```python
from build123d import *

# Parameters (mm, degrees)
F0_W     = 508
F0_H     = 508
F1_DEPTH = 15.875
F4_R     = 12.7
F5_R     = 12.7
F6_R     = 12.7


# Not quite as in the source:
# - the program builds the solid bodies; features that only make, move or delete a surface that nothing else refers to are left out


with BuildPart() as f1:
    # F0 (on Top) → F1 (new body)
    with BuildSketch(Plane.XY):
        with Locations((-1.661028713, -10.90797159)):
            Rectangle(F0_W, F0_H)
    extrude(amount=F1_DEPTH)

    # F4
    f4_edges = [f1.edges().sort_by_distance(p)[0] for p in [
        (252.338971, 243.092028, 7.9375),
        (252.338971, -264.907972, 7.9375),
    ]]
    fillet(f4_edges, radius=F4_R)

    # F5
    f5_edges = [f1.edges().sort_by_distance(p)[0] for p in [
        (-255.661029, 243.092028, 7.9375),
        (-255.661029, -264.907972, 7.9375),
    ]]
    fillet(f5_edges, radius=F5_R)

    # F6
    f6_edges = [f1.edges().sort_by_distance(p)[0] for p in [
        (-1.661029, 243.092028, 15.875),
        (-251.941285, 239.372285, 15.875),
        (248.619227, 239.372285, 15.875),
        (-255.661029, -10.907972, 15.875),
        (252.338971, -10.907972, 15.875),
        (-251.941285, -261.188228, 15.875),
        (248.619227, -261.188228, 15.875),
        (-1.661029, -264.907972, 15.875),
    ]]
    fillet(f6_edges, radius=F6_R)


solid = f1.part
```
Could you check a few things on this model? Use its own coordinates, in mm. Round coordinates to 2 decimals unless told otherwise and drop trailing zeros. Loops run counter-clockwise (first coordinate to the right, second up) from the corner with the lowest first, then second, coordinate; pieces in that order, holes last.
Q1. Please list where these lines run through material, in increasing order: L1, parallel to X at y = 80, z = 3.75; L2, parallel to Y at x = -177.5, z = 4; L3, parallel to X at y = -158, z = 7.5.
Q2. For P1, Ø1, axis at x = -93, z = 11.5, coming from the +Y side (3 decimals); P2, Ø8, axis at x = -38.5, z = 14, coming from the +Y side; P3, Ø5, axis at y = 120.5, z = 11, coming from the -X side, each with a flat end and sliding along its axis, tell me the tip position at first contact or that it passes through.
Q3. I want a section at A-A (z = 13.25). Write out the boundary of the cut face in (x, y).
Answer below:
1. L1: x = -255.65 to 252.33
1. L2: y = -264.88 to 243.07
1. L3: x = -254.9 to 251.58
2. P1: stops at y = 240.395
2. P2: stops at y = 241.1
2. P3: stops at x = -254.49
3. outline: (-250.69, -252.21) arc R7.73 ccw to (-242.96, -259.94) - (239.64, -259.94) arc R7.73 ccw to (247.37, -252.21) - (247.37, 230.39) arc R7.73 ccw to (239.64, 238.12) - (-242.96, 238.12) arc R7.73 ccw to (-250.69, 230.39) - close
